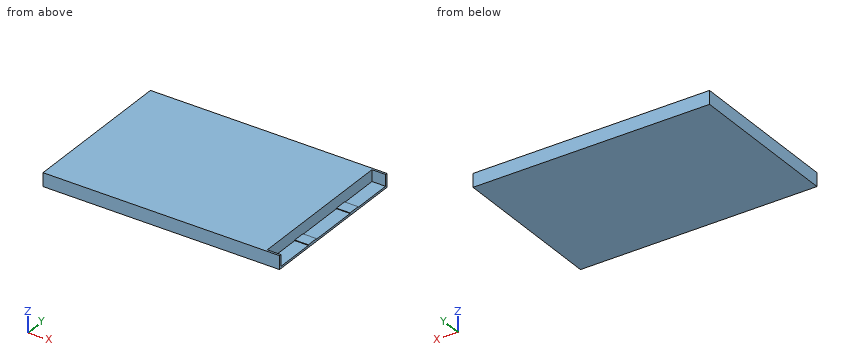
from build123d import *

# Parameters (mm, degrees)
SKETCH1_W           = 100.33
SKETCH1_H           = 67.31
BOSS_EXTRUDE1_DEPTH = 2.8575
SKETCH2_W           = 5.7912
SKETCH2_H           = 65.5828
CUT_EXTRUDE1_DEPTH  = 4.8514
SKETCH3_W           = 5.7912
SKETCH3_H           = 5.08
BOSS_EXTRUDE2_DEPTH = 0.254


with BuildPart() as part:
    # Sketch1 → Boss-Extrude1 (new, symmetric)
    with BuildSketch(Plane.XY):
        Rectangle(SKETCH1_W, SKETCH1_H)
    extrude(amount=BOSS_EXTRUDE1_DEPTH, both=True)

    # Sketch2 → Cut-Extrude1 (cut)
    with BuildSketch(Plane.XY.offset(2.8575)):
        with Locations((47.2694, 0)):
            Rectangle(SKETCH2_W, SKETCH2_H)
    extrude(amount=-CUT_EXTRUDE1_DEPTH, mode=Mode.SUBTRACT)

    # Sketch3 → Boss-Extrude2 (add)
    with BuildSketch(Plane.XY.offset(-1.9939)):
        with Locations((47.2694, -13.0556)):
            Rectangle(SKETCH3_W, SKETCH3_H)
        with Locations((47.2694, 13.0556)):
            Rectangle(SKETCH3_W, SKETCH3_H)
    extrude(amount=BOSS_EXTRUDE2_DEPTH)


solid = part.part
The listing builds one solid part. Answer for the finished solid, in the listing's coordinates (mm). Give positions to 0.01 mm unless a question says otherwise; leave off trailing zeros. Write each loop counter-clockwise with the first axis right and the second up, starting at its lowest first coordinate (ties: lowest second). Pieces come first, ordered by that corner, then holes.
Item 1: Find the intervals of material crossed by line 1 along X through (y, z) = (-22.5, 1.1) (3 decimals), in increasing order.
Item 2: Flat-ended cylindrical pins translate along their axes: P1, Ø4.5, axis at x = 48.5, y = -1.5, coming from the +Z side; P2, Ø5.5, axis at x = 48, y = -13, coming from the +Z side; P3, Ø1.5, axis at y = 14.5, z = 0, coming from the +X side. Find the tip coordinate at first contact, or state that the pin passes through.
Item 3: Section C-C, the plane y = -1 is taken. Write down the section's boundary in (x, z) (1 decimal), plus the area to 3 significant figures.
Item 4: Section A-A, the plane y = 12.5 is taken. Write down the section's boundary in (x, z) (1 decimal).
Item 5: Section B-B, the plane z = 1.45 is taken. Write down the section's boundary in (x, y) (3 decimals).
Completed:
1. line 1: x = -50.165 to 44.374
2. P1: stops at z = -1.99
2. P2: stops at z = -1.74
2. P3: stops at x = 44.37
3. outline: (-50.2, -2.9) - (50.2, -2.9) - (50.2, -2) - (44.4, -2) - (44.4, 2.9) - (-50.2, 2.9) - close
3. area: 545 mm2
4. outline: (-50.2, -2.9) - (50.2, -2.9) - (50.2, -1.7) - (44.4, -1.7) - (44.4, 2.9) - (-50.2, 2.9) - close
5. outline: (-50.165, -33.655) - (50.165, -33.655) - (50.165, -32.791) - (44.374, -32.791) - (44.374, 32.791) - (50.165, 32.791) - (50.165, 33.655) - (-50.165, 33.655) - close
